```python
from build123d import *

# Parameters (mm, degrees)
SKETCH1_W           = 23.876
SKETCH1_H           = 9.525
SKETCH1_R           = 1.778
BOSS_EXTRUDE1_DEPTH = 6
CUT_EXTRUDE3_DEPTH  = 15.184401653
FILLET1_R           = 0.3048


with BuildPart() as part:
    # Sketch1 → Boss-Extrude1 (new body)
    with BuildSketch(Plane.XY):
        Rectangle(SKETCH1_W, SKETCH1_H)
        Circle(SKETCH1_R, mode=Mode.SUBTRACT)
    extrude(amount=BOSS_EXTRUDE1_DEPTH)

    # Sketch2 → Cut-Extrude3 (cut, through all)
    with BuildSketch(Plane.XY.offset(6)):
        Polygon((-11.938, -0.4572), (-3.81, -0.4572), (-3.81, 0), (-3.81, 0.254), (-3.976407191, 0.7112), (-4.826, 0.7112), (-4.992407191, 0.254), (-5.842, 0.254), (-6.008407191, 0.7112), (-6.858, 0.7112), (-7.024407191, 0.254), (-7.874, 0.254), (-8.040407191, 0.7112), (-8.89, 0.7112), (-9.056407191, 0.254), (-9.906, 0.254), (-10.072407191, 0.7112), (-10.922, 0.7112), (-11.088407191, 0.254), (-11.938, 0.254), align=None)
        Polygon((-11.938, 4.7625), (-11.938, 2.2225), (-3.048, 4.7625), align=None)
        Polygon((-11.938, -2.2225), (-11.938, -4.7625), (-3.048, -4.7625), align=None)
    cut_extrude3 = extrude(amount=-CUT_EXTRUDE3_DEPTH, mode=Mode.SUBTRACT)

    # Mirror1: Cut-Extrude3 across plane
    add(cut_extrude3.mirror(Plane(origin=(0, 0, 0), x_dir=(0, 0, 1), z_dir=(1, 0, 0))), mode=Mode.SUBTRACT)

    # Fillet1
    fillet1_edges = [part.edges().sort_by_distance(p)[0] for p in [
        (4.992407191, 0.254, 3),
        (5.842, 0.254, 3),
        (7.024407191, 0.254, 3),
        (7.874, 0.254, 3),
        (9.056407191, 0.254, 3),
        (9.906, 0.254, 3),
        (11.088407191, 0.254, 3),
        (3.048, 4.7625, 3),
        (11.938, 2.2225, 3),
        (3.048, -4.7625, 3),
        (11.938, -2.2225, 3),
        (-11.088407191, 0.254, 3),
        (-9.906, 0.254, 3),
        (-9.056407191, 0.254, 3),
        (-7.874, 0.254, 3),
        (-7.024407191, 0.254, 3),
        (-5.842, 0.254, 3),
        (-4.992407191, 0.254, 3),
        (-3.048, 4.7625, 3),
        (-11.938, 2.2225, 3),
        (-11.938, -2.2225, 3),
        (-3.048, -4.7625, 3),
    ]]
    fillet(fillet1_edges, radius=FILLET1_R)


solid = part.part
```
The listing builds one solid part. Answer for the finished solid, in the listing's coordinates (mm). A direction names the side the tool comes from. Give positions to 0.01 mm unless a question says otherwise; leave off trailing zeros. Order: outer loops, then holes, each group sorted by start corner. A loop starts at its lowest first (then second) coordinate and runs counter-clockwise, first axis right, second up. Notation, with made-up numbers: M 46.25,78.5 L 66.25,78.5 A18 cw 66.25,96.5 Z; hole C 21,35.5 d7. An arc over 180 degrees is marked long. Put each result on its own line as item: value. Start each with the question number.
Item 1: Flat-ended cylindrical pins translate along their axes: P1, Ø0.7, axis at x = -4.5, z = 2, coming from the -Y side; P2, Ø0.9, axis at x = -8.5, z = 4, coming from the -Y side; P3, Ø0.7, axis at x = -10.5, z = 2.5, coming from the -Y side. Find the tip coordinate at first contact, or state that the pin passes through.
Item 2: For a pull along Y with two mould halves and no side action, classify faces 4 (the face through (0, -2, 6)), 5 (the face through (-7.343, -3.535, 3.042)), 6 (the face through (-8, -0.457, 3)), 7 (the face through (6.4, 0.711, 3)) as +Y half, -Y half, draft (parallel to the pull), parting line (faces both ways), or undercut.
Item 3: The part is cut by section B-B, the plane x = 0. Determine the outline of the cut face in (y, z), and give its area (3 significant figures).
Item 4: The part is cut by section D-D, the plane y = -4. Determine the outline of the cut face in (x, z).
Item 5: The part is cut by section C-C, the plane y = 3.5. Determine the outline of the cut face in (x, z), and give its area (3 significant figures).
Item 6: The part is cut by section A-A, the plane y = 0. Determine the outline of the cut face in (x, z).
Item 7: Find the intervals of material crossed by line 1 along Y through (x, z) = (0, 1.3); line 2 along Y through (x, z) = (-5, 4.6); line 3 along X through (y, z) = (2.25, 3.15), in increasing order.
Item 8: Which of the six approach directions +Z, -Z, +X, -X, +Y, -Y give full straight-line access (tool end or side, diameter ignored) to faces 1 (the face through (8.5, 0.711, 3)), 2 (the face through (8, -0.457, 3)), 3 (the face through (-7.46, 3.5, 3.04))?
Answer key:
1. P1: stops at y = -4.45
1. P2: stops at y = -3.33
1. P3: stops at y = -2.73
2. face 4: draft
2. face 5: -Y half
2. face 6: undercut
2. face 7: undercut
3. outline: M -4.76,0 L -1.78,0 L -1.78,6 L -4.76,6 Z; M 1.78,0 L 4.76,0 L 4.76,6 L 1.78,6 Z
3. area: 35.8 mm²
4. outline: M -5.72,0 L 5.72,0 L 5.72,6 L -5.72,6 Z
5. outline: M -7.47,0 L 7.47,0 L 7.47,6 L -7.47,6 Z
5. area: 89.6 mm²
6. outline: M -3.81,0 L -1.78,0 L -1.78,6 L -3.81,6 Z; M 1.78,0 L 3.81,0 L 3.81,6 L 1.78,6 Z
7. line 1: y = -4.76 to -1.78, 1.78 to 4.76
7. line 2: y = -4.2 to -0.46, 0.33 to 4.2
7. line 3: x = -11.8 to 11.8
8. face 1: +Z, -Z
8. face 2: +Z, -Z, +X
8. face 3: +Z, -Z, -X, +Y
